The figure shows three views and two pictorial views of one solid part (mm, origin at its lowest corner). Answer the questions. Coordinates: 2 decimals unless noted, no trailing zeros. Order: outer loops, then holes, each group sorted by start corner. A loop starts at its lowest first (then second) coordinate and runs counter-clockwise, first axis right, second up. Notation, with made-up numbers: (53.5, 57) -> (68.5, 57) arc R25 cw to (68.5, 75) -> close; hole circle Ø2 at (35, -31.75). An arc over 180 degrees is marked (long way). Use one line per item in the form item = value.
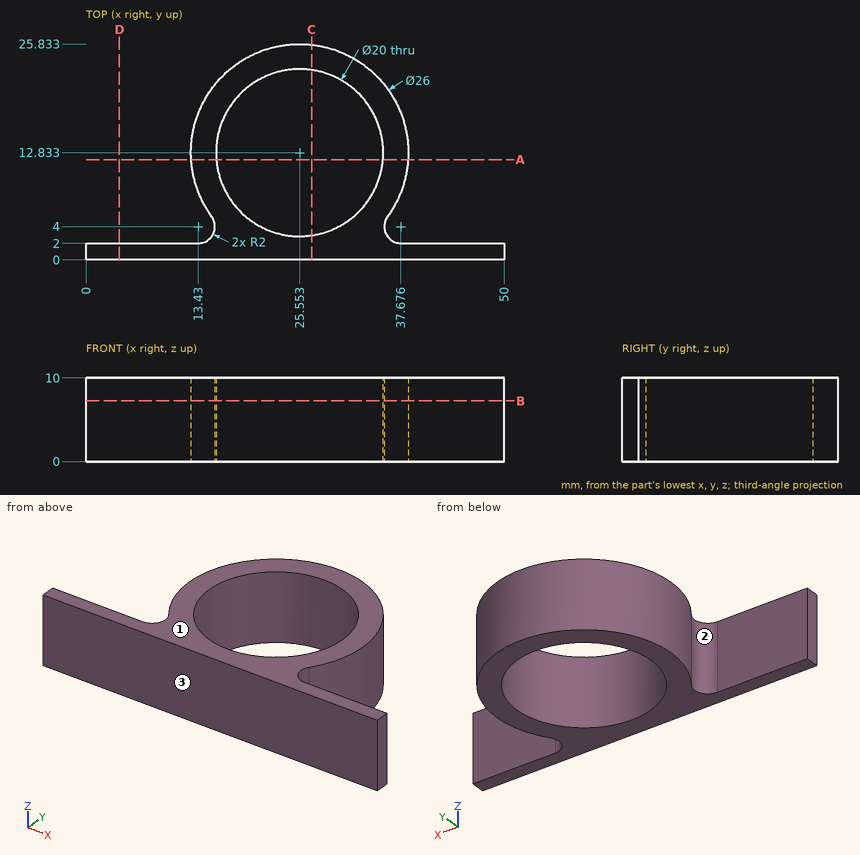
(1) Section A-A on y = 12 is taken. Write down the section's boundary in (x, z).
Data:
outline = (12.58, 0) -> (15.59, 0) -> (15.59, 10) -> (12.58, 10) -> close; (35.52, 0) -> (38.53, 0) -> (38.53, 10) -> (35.52, 10) -> close
(2) The mould has two halves that part along Y. Classify the marked faces 1, 2 and 3: released by +Y, released by -Y, zero draft, split by the parting line, or undercut.
Data:
face_1 = zero draft
face_2 = undercut
face_3 = released by -Y
(3) Straight lines are drawn through the part: line 1 along Y through (x, z) = (25.5, 8.75); line 2 along Y through (x, z) = (19, 7.5) (1 decimal); line 3 along X through (y, z) = (12.75, 7). For each, find the intervals that lie inside material, in ascending order.
Data:
line_1 = 0 to 2.83, 22.83 to 25.83
line_2 = 0 to 5.3, 20.4 to 24.1
line_3 = 12.55 to 15.55, 35.55 to 38.55
(4) Each of these flat-tipped pins is pushed along its axis until it touches: P1, Ø5, axis at y = 14, z = 3.5, coming from the -X side; P2, Ø6, axis at x = 33, z = 3, coming from the +Y side; P3, Ø1.5, axis at y = 7.5, z = 5.5, coming from the -X side; P4, Ø2, axis at x = 11.5, y = 12.5, coming from the +Z side. Where does it stop, or does it pass through?
Data:
P1 = 12.55
P2 = 25.05
P3 = 13.39
P4 = through
(5) Section C-C on x = 27 is taken. Write down the section's boundary in (y, z).
Data:
outline = (0, 0) -> (2.94, 0) -> (2.94, 10) -> (0, 10) -> close; (22.73, 0) -> (25.75, 0) -> (25.75, 10) -> (22.73, 10) -> close
(6) Section D-D on x = 4 is taken. Write down the section's boundary in (y, z).
Data:
outline = (0, 0) -> (2, 0) -> (2, 10) -> (0, 10) -> close
(7) Section B-B on z = 7.25 is taken. Write down the section's boundary in (x, y).
Data:
outline = (0, 0) -> (50, 0) -> (50, 2) -> (37.68, 2) arc R2 cw to (36.06, 5.18) arc R13 ccw (long way) to (15.05, 5.18) arc R2 cw to (13.43, 2) -> (0, 2) -> close; hole circle Ø20 at (25.55, 12.83)
